from build123d import *

# Parameters (mm, degrees)
BOSS_EXTRUDE1_DEPTH = 10


with BuildPart() as part:
    # Sketch1 → Boss-Extrude1 (new body)
    with BuildSketch(Plane.XY):
        with BuildLine():
            Line((6.747131567, 0), (57.259771997, 0))
            ThreePointArc((57.259771997, 0), (59.570856854, 0.673619806), (61.158070395, 2.483489977))
            Line((61.158070395, 2.483489977), (75.800845312, 33.885022121))
            ThreePointArc((75.800845312, 33.885022121), (75.530405908, 38.011130086), (71.90517476, 40))
            Line((71.90517476, 40), (21.392534329, 40))
            ThreePointArc((21.392534329, 40), (19.081449472, 39.326380194), (17.494235931, 37.516510023))
            Line((17.494235931, 37.516510023), (2.851461014, 6.114977879))
            ThreePointArc((2.851461014, 6.114977879), (3.121900418, 1.988869914), (6.747131567, 0))
        make_face()
        with BuildLine():
            ThreePointArc((4.210922695, 5.481050486), (4.386987587, 2.794819326), (6.747131567, 1.5))
            Line((6.747131567, 1.5), (57.259771997, 1.5))
            ThreePointArc((57.259771997, 1.5), (58.764907442, 1.938706975), (59.798608715, 3.11741737))
            Line((59.798608715, 3.11741737), (74.441383631, 34.518949514))
            ThreePointArc((74.441383631, 34.518949514), (74.265318739, 37.205180674), (71.90517476, 38.5))
            Line((71.90517476, 38.5), (21.392534329, 38.5))
            ThreePointArc((21.392534329, 38.5), (19.887398884, 38.061293025), (18.853697612, 36.88258263))
            Line((18.853697612, 36.88258263), (4.210922695, 5.481050486))
        make_face(mode=Mode.SUBTRACT)
    extrude(amount=BOSS_EXTRUDE1_DEPTH)


solid = part.part
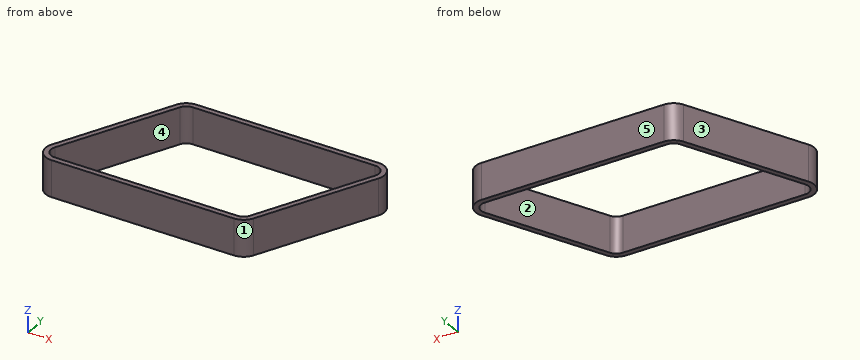
For this review, take the finished solid that the model builds, in its own axes (mm). Face numbers are marked on the shaded views. A direction names the side the tool comes from. Round coordinates to 2 decimals unless told otherwise and drop trailing zeros. Write each loop counter-clockwise with the first axis right and the second up, starting at its lowest first coordinate (ties: lowest second). Pieces come first, ordered by that corner, then holes. Notation, with made-up numbers: (17.5, 70.5) - (36.5, 70.5) arc R31 cw to (36.5, 97.5) - close; hole circle Ø2 at (67.25, 58). An arc over 180 degrees is marked (long way). Write item = value, one per line. Start each with the question number.
1. Consider section C-C on y = 16. State the section outline as (x, z) points.
2. Consider section A-A on x = 28. State the section outline as (y, z) points, plus the area to 3 significant figures.
3. For the marked faces 4 and 5, list the 3-axis set-ups (+Z, -Z, +X, -X, +Y, -Y) from which the entire face can be reached by the end or side of a thin tool; tool diameter is ignored.
4. For pin 1 Ø6 at (y, z) = (8, 2) entering from -X; pin 2 Ø3 at (x, y) = (62, 10.5) entering from -Z; pin 3 Ø1.5 at (y, z) = (34.5, 4) entering from +X; pin 4 Ø2 at (y, z) = (32.5, 5) entering from +X, all flat-tipped, find the tip position at first contact; note any pin that passes through.
5. Wall thickness on L1, parallel to Y at x = 30.5, z = 8; L2, parallel to X at y = 29.5, z = 1.5; L3, parallel to X at y = 10.5, z = 1.5: over which ranges is each line inside the solid? List them lowest first.
6. Draft analysis for pull direction Y (two halves, no side actions). For the marked faces 1, 2 and 3, state which applies: released by +Y, released by -Y, zero draft, split by the parting line, or undercut.
7. Consider section B-B on z = 6.75. State the section outline as (x, y) points, plus the area to 3 significant figures.
Evaluation:
q1.outline = (7.46, 0) - (9.12, 0) - (9.12, 10) - (7.46, 10) - close; (65.81, 0) - (67.46, 0) - (67.46, 10) - (65.81, 10) - close
q2.outline = (0, 0) - (1.5, 0) - (1.5, 10) - (0, 10) - close; (38.5, 0) - (40, 0) - (40, 10) - (38.5, 10) - close
q2.area = 30.0 mm2
q3.face_4 = +Z, -Z
q3.face_5 = +Z, -Z, +X, -X, +Y
q4.pin_1 = 2.51
q4.pin_2 = 0
q4.pin_3 = 76.18
q4.pin_4 = 75.62
q5.L1 = 0 to 1.5, 38.5 to 40
q5.L2 = 13.76 to 15.41, 72.1 to 73.76
q5.L3 = 4.9 to 6.55, 63.24 to 64.9
q6.face_1 = released by -Y
q6.face_2 = undercut
q6.face_3 = released by +Y
q7.outline = (2.85, 6.11) arc R4.3 ccw to (6.75, 0) - (57.26, 0) arc R4.3 ccw to (61.16, 2.48) - (75.8, 33.89) arc R4.3 ccw to (71.91, 40) - (21.39, 40) arc R4.3 ccw to (17.49, 37.52) - close; hole (4.21, 5.48) arc R2.8 ccw to (6.75, 1.5) - (57.26, 1.5) arc R2.8 ccw to (59.8, 3.12) - (74.44, 34.52) arc R2.8 ccw to (71.91, 38.5) - (21.39, 38.5) arc R2.8 ccw to (18.85, 36.88) - close
q7.area = 289 mm2
